Geometry check sheet. Reference: the model listing, model coordinates, mm. Coordinates: 2 decimals unless noted, no trailing zeros. Write each loop counter-clockwise with the first axis right and the second up, starting at its lowest first coordinate (ties: lowest second). Pieces come first, ordered by that corner, then holes. Notation, with made-up numbers: (-15, 62.25) -> (17, 62.25) arc R34 ccw to (17, 101.25) -> close; hole circle Ø1 at (-37.5, 19.5). An arc over 180 degrees is marked (long way). Put each result on its own line as item: value. Start each with the question number.
from build123d import *

# Parameters (mm, degrees)
SKETCH1_R           = 56
SKETCH1_R_2         = 2
SKETCH1_R_3         = 2.5
BOSS_EXTRUDE1_DEPTH = 4
SKETCH4_R           = 8.5
CUT_EXTRUDE2_DEPTH  = 171.674300953
SKETCH6_R           = 8.5
CUT_EXTRUDE4_DEPTH  = 171.674300953
SKETCH7_R           = 2.5
CUT_EXTRUDE5_DEPTH  = 171.674300953
BOSS_EXTRUDE3_DEPTH = 4


with BuildPart() as part:
    # Sketch1 → Boss-Extrude1 (new body)
    with BuildSketch(Plane.XY):
        with BuildLine():
            Line((-112.067145126, 20.879542552), (-112.067145126, -35.368944903))
            ThreePointArc((-112.067145126, -35.368944903), (-109.233115964, -42.343818518), (-102.337372736, -45.365293088))
            Line((-102.337372736, -45.365293088), (-53.565458311, -46.683726342))
            ThreePointArc((-53.565458311, -46.683726342), (-39.773971855, -52.726675482), (-34.105913531, -66.676422713))
            Line((-34.105913531, -66.676422713), (-34.105913531, -118.664960222))
            ThreePointArc((-34.105913531, -118.664960222), (-31.176981342, -125.736028034), (-24.105913531, -128.664960222))
            Line((-24.105913531, -128.664960222), (58.614189281, -128.664960222))
            Line((58.614189281, -128.664960222), (88.614189281, -128.664960222))
            ThreePointArc((88.614189281, -128.664960222), (92.149723187, -127.200494128), (93.614189281, -123.664960222))
            Line((93.614189281, -123.664960222), (93.614189281, 90.572680082))
            ThreePointArc((93.614189281, 90.572680082), (92.149723187, 94.108213988), (88.614189281, 95.572680082))
            Line((88.614189281, 95.572680082), (58.614189281, 95.572680082))
            Line((58.614189281, 95.572680082), (-0.097235187, 95.572680082))
            Line((-0.097235187, 95.572680082), (-102.067145126, 95.572680082))
            ThreePointArc((-102.067145126, 95.572680082), (-109.138212938, 92.643747894), (-112.067145126, 85.572680082))
            Line((-112.067145126, 85.572680082), (-112.067145126, 20.879542552))
        make_face()
        Circle(SKETCH1_R, mode=Mode.SUBTRACT)
        with Locations((-90.866128835, 53.212776201)):
            Circle(SKETCH1_R_2, mode=Mode.SUBTRACT)
        with Locations((60.411582215, 53.410160046)):
            Circle(SKETCH1_R_2, mode=Mode.SUBTRACT)
        with Locations((68.053955118, -43.027190126)):
            Circle(SKETCH1_R_2, mode=Mode.SUBTRACT)
        with Locations((-70.733552477, -41.68716468)):
            Circle(SKETCH1_R_2, mode=Mode.SUBTRACT)
        with Locations((29.113560385, -56.573326106)):
            Circle(SKETCH1_R_3, mode=Mode.SUBTRACT)
        with Locations((-106.987586177, -23.437423897)):
            Circle(SKETCH1_R_2, mode=Mode.SUBTRACT)
        with Locations((-106.333483393, 26.197806711)):
            Circle(SKETCH1_R_2, mode=Mode.SUBTRACT)
        with Locations((-97.118043766, 84.840447035)):
            Circle(SKETCH1_R_3, mode=Mode.SUBTRACT)
        with Locations((82.881956234, -115.159552965)):
            Circle(SKETCH1_R_3, mode=Mode.SUBTRACT)
        with Locations((-56.573326106, -29.113560385)):
            Circle(SKETCH1_R_3, mode=Mode.SUBTRACT)
        with Locations((-29.113560385, 56.573326106)):
            Circle(SKETCH1_R_3, mode=Mode.SUBTRACT)
        with Locations((56.573326106, 29.113560385)):
            Circle(SKETCH1_R_3, mode=Mode.SUBTRACT)
        with Locations((-47.118043766, 84.840447035)):
            Circle(SKETCH1_R_3, mode=Mode.SUBTRACT)
        with Locations((2.881956234, 84.840447035)):
            Circle(SKETCH1_R_3, mode=Mode.SUBTRACT)
        with Locations((52.881956234, 84.840447035)):
            Circle(SKETCH1_R_3, mode=Mode.SUBTRACT)
        with Locations((82.881956234, -59.119552965)):
            Circle(SKETCH1_R_3, mode=Mode.SUBTRACT)
        with Locations((82.881956234, -3.079552965)):
            Circle(SKETCH1_R_3, mode=Mode.SUBTRACT)
        with Locations((82.881956234, 52.960447035)):
            Circle(SKETCH1_R_3, mode=Mode.SUBTRACT)
    extrude(amount=BOSS_EXTRUDE1_DEPTH)

    # Sketch4 → Cut-Extrude2 (cut, through all)
    with BuildSketch(Plane(origin=(0, 0, 0), x_dir=(-1, 0, 0), z_dir=(0, 0, -1))):
        with Locations((-24.413036242, -94.796918523)):
            Circle(SKETCH4_R)
    extrude(amount=-CUT_EXTRUDE2_DEPTH, mode=Mode.SUBTRACT)

    # Sketch6 → Cut-Extrude4 (cut, through all)
    with BuildSketch(Plane.XY.offset(4)):
        with Locations((-78.790468385, 2.794224701)):
            Circle(SKETCH6_R)
    extrude(amount=-CUT_EXTRUDE4_DEPTH, mode=Mode.SUBTRACT)

    # Sketch7 → Cut-Extrude5 (cut, through all)
    with BuildSketch(Plane.XY.offset(4)):
        with Locations((42.373548484, -76.836406281)):
            Circle(SKETCH7_R)
        with Locations((6.452523999, -112.757430765)):
            Circle(SKETCH7_R)
        with Locations((6.452523999, -76.836406281)):
            Circle(SKETCH7_R)
        with Locations((42.373548484, -112.757430765)):
            Circle(SKETCH7_R)
    extrude(amount=-CUT_EXTRUDE5_DEPTH, mode=Mode.SUBTRACT)

    # Sketch8 → Boss-Extrude3 (add)
    with BuildSketch(Plane.XY.offset(4)):
        with BuildLine():
            Line((-52.172571307, -46.669291865), (-39.028626082, -47.635255681))
            Line((-39.028626082, -47.635255681), (-0.218247557, -69.999659771))
            ThreePointArc((-0.218247557, -69.999659771), (-28.675355133, -63.857059187), (-52.172571307, -46.669291865))
        make_face()
    extrude(amount=-BOSS_EXTRUDE3_DEPTH)


solid = part.part
Item 1: Scan lines: line 1 along Y through (x, z) = (83, 2.95); line 2 along X through (y, z) = (-77, 3.1); line 3 along Y through (x, z) = (27.5, 2). Record each from-to range of solid material in increasing order. Write a range as [from, to].
Item 2: Section check B-B, the plane z = 1.95. Give the number of separate pieces and of enclosed holes in the cut face, and give its area (3 significant figures).
Item 3: Section check A-A, the plane x = -17.5. Enter the section's corners in (y, z), and give its area (3 significant figures).
Item 4: Section check C-C, the plane x = -63.5. Enter the section's corners in (y, z), and give its area (3 significant figures).
Item 5: Mould release check, pull along Y, two halves, no side actions. Record for faces 1 (the cylindrical face through (51.73, -21.45, 1.97)), 2 (the cylindrical face through (92.19, 94.07, 1.97)), 3 (the flat face through (-56, -15, 0)): released by +Y, released by -Y, zero draft, split by the parting line, or undercut.
Item 6: Go/stop test with flat-tipped pins: P1, Ø1.5, axis at y = -80, z = 2, coming from the -X side; P2, Ø8, axis at x = -97.12, y = 84.84, coming from the -Z side. Record where each tip stops, or that it passes through.
From the geometry:
1. line 1: [-128.66, -117.66], [-112.66, -61.62], [-56.62, -5.58], [-0.58, 50.46], [55.46, 95.57]
1. line 2: [-34.11, 3.96], [8.95, 39.88], [44.87, 93.61]
1. line 3: [-128.66, -102.72], [-86.88, -58.48], [-54.66, -48.78], [48.78, 95.57]
2. separate pieces: 1
2. enclosed holes: 25
2. area: 29,100 mm²
3. outline: (-128.66, 0) -> (-53.2, 0) -> (-53.2, 4) -> (-128.66, 4) -> close; (53.2, 0) -> (95.57, 0) -> (95.57, 4) -> (53.2, 4) -> close
3. area: 471 mm²
4. outline: (-46.42, 0) -> (95.57, 0) -> (95.57, 4) -> (-46.42, 4) -> close
4. area: 568 mm²
5. face 1: undercut
5. face 2: released by +Y
5. face 3: zero draft
6. P1: x = -34.11
6. P2: z = 0
